from build123d import *

# Parameters (mm, degrees)
SKETCH1_W               = 203.2
SKETCH1_H               = 203.2
BOSS_EXTRUDE1_DEPTH     = 6.35
SKETCH2_W               = 44.45
SKETCH2_H               = 45.72
SKETCH2_H_2             = 50.8
CUT_EXTRUDE1_DEPTH      = 144.824345992
SKETCH3_R               = 2.54
SKETCH3_W               = 25.4
SKETCH3_H               = 25.4
CUT_EXTRUDE2_DEPTH      = 6.35
MIRROR2_COPY_1_SKETCH_R = 2.54
MIRROR2_COPY_1_SKETCH_W = 25.4
MIRROR2_COPY_1_SKETCH_H = 25.4
MIRROR2_COPY_1_DEPTH    = 6.35
SKETCH4_W               = 101.6
SKETCH4_H               = 93.98
SKETCH4_W_2             = 95.25
SKETCH4_H_2             = 87.63
BOSS_EXTRUDE2_DEPTH     = 152.4
SKETCH5_W               = 10
SKETCH5_H               = 10
SKETCH5_R               = 1.6
BOSS_EXTRUDE3_DEPTH     = 3.175
CUT_EXTRUDE3_REACH      = 246.393
SKETCH8_R               = 1.905
SKETCH9_W               = 6.35
SKETCH9_H               = 152.4
BOSS_EXTRUDE4_DEPTH     = 44.45
SKETCH12_W              = 3.175
SKETCH12_H              = 3.81
CUT_EXTRUDE4_DEPTH      = 152.4
SKETCH13_W              = 38.1
SKETCH13_H              = 3.81
CUT_EXTRUDE5_DEPTH      = 3.175
SKETCH14_W              = 6.35
SKETCH14_H              = 152.4
BOSS_EXTRUDE5_DEPTH     = 44.45
SKETCH15_W              = 3.175
SKETCH15_H              = 3.81
CUT_EXTRUDE6_DEPTH      = 152.4
SKETCH16_W              = 38.1
SKETCH16_H              = 3.81
CUT_EXTRUDE7_DEPTH      = 3.175
CUT_EXTRUDE8_REACH      = 211.454
SKETCH17_R              = 6.35
MIRROR5_OUTLINE_R       = 6.35
MIRROR5_DEPTH           = 6.35


# Read off the part's stored shape, not the designer's step: Mirror5
with BuildPart() as part:
    # Sketch1 → Boss-Extrude1 (new body)
    with BuildSketch(Plane(origin=(0, 0, 0), x_dir=(1, 0, 0), z_dir=(0, 1, 0))):
        Rectangle(SKETCH1_W, SKETCH1_H)
    extrude(amount=BOSS_EXTRUDE1_DEPTH)

    # Sketch2 → Cut-Extrude1 (cut, through all)
    with BuildSketch(Plane(origin=(0, 6.35, 0), x_dir=(1, 0, 0), z_dir=(0, 1, 0))):
        with Locations((0, 78.74)):
            Rectangle(SKETCH2_W, SKETCH2_H)
        with Locations((0, -76.2)):
            Rectangle(SKETCH2_W, SKETCH2_H_2)
    extrude(amount=-CUT_EXTRUDE1_DEPTH, mode=Mode.SUBTRACT)

    # Sketch3 → Cut-Extrude2 (cut)
    with BuildSketch(Plane(origin=(0, 6.35, 0), x_dir=(1, 0, 0), z_dir=(0, 1, 0))):
        with Locations(Location((-96.52, 76.2, 0), (0, 0, 270))):
            Circle(SKETCH3_R)
        with Locations(Location((-76.2, 96.52, 0), (0, 0, 270))):
            Circle(SKETCH3_R)
        with Locations(Location((-76.2, 55.88, 0), (0, 0, 270))):
            Circle(SKETCH3_R)
        with Locations(Location((-41.275, 96.52, 0), (0, 0, 270))):
            Circle(SKETCH3_R)
        with Locations(Location((-41.275, 55.88, 0), (0, 0, 90))):
            Circle(SKETCH3_R)
        with Locations((-41.148, 76.2)):
            Rectangle(SKETCH3_W, SKETCH3_H)
        with Locations((-76.2, 76.2)):
            Rectangle(SKETCH3_W, SKETCH3_H)
    cut_extrude2 = extrude(amount=-CUT_EXTRUDE2_DEPTH, mode=Mode.SUBTRACT)

    # Mirror1: Cut-Extrude2 across plane
    add(cut_extrude2.mirror(Plane(origin=(0, 0, 0), x_dir=(0, 0, 1), z_dir=(1, 0, 0))), mode=Mode.SUBTRACT)

    # Mirror2: Cut-Extrude2 across plane
    add(cut_extrude2.mirror(Plane.XY), mode=Mode.SUBTRACT)

    # Mirror2 copy 1 sketch → Mirror2 copy 1 (cut)
    with BuildSketch(Plane(origin=(0, 6.35, 0), x_dir=(-1, 0, 0), z_dir=(0, 1, 0))):
        with Locations(Location((-96.52, 76.2, 0), (0, 0, 270))):
            Circle(MIRROR2_COPY_1_SKETCH_R)
        with Locations(Location((-76.2, 96.52, 0), (0, 0, 270))):
            Circle(MIRROR2_COPY_1_SKETCH_R)
        with Locations(Location((-76.2, 55.88, 0), (0, 0, 270))):
            Circle(MIRROR2_COPY_1_SKETCH_R)
        with Locations(Location((-41.275, 96.52, 0), (0, 0, 270))):
            Circle(MIRROR2_COPY_1_SKETCH_R)
        with Locations(Location((-41.275, 55.88, 0), (0, 0, 90))):
            Circle(MIRROR2_COPY_1_SKETCH_R)
        with Locations((-41.148, 76.2)):
            Rectangle(MIRROR2_COPY_1_SKETCH_W, MIRROR2_COPY_1_SKETCH_H)
        with Locations((-76.2, 76.2)):
            Rectangle(MIRROR2_COPY_1_SKETCH_W, MIRROR2_COPY_1_SKETCH_H)
    extrude(amount=-MIRROR2_COPY_1_DEPTH, mode=Mode.SUBTRACT)

    # Sketch4 → Boss-Extrude2 (add)
    with BuildSketch(Plane(origin=(0, 6.35, 0), x_dir=(1, 0, 0), z_dir=(0, 1, 0))):
        with Locations((0, 2.54)):
            Rectangle(SKETCH4_W, SKETCH4_H)
        with Locations((0, 2.54)):
            Rectangle(SKETCH4_W_2, SKETCH4_H_2, mode=Mode.SUBTRACT)
    extrude(amount=BOSS_EXTRUDE2_DEPTH)

    # Sketch5 → Boss-Extrude3 (add)
    # profile 1 of 4: a face of its own
    with BuildSketch(Plane(origin=(50.8, 0, 0), x_dir=(0, 0, -1), z_dir=(1, 0, 0))):
        with Locations((-21.59, 93.98)):
            Rectangle(SKETCH5_W, SKETCH5_H)
        with Locations((-21.59, 93.98)):
            Circle(SKETCH5_R, mode=Mode.SUBTRACT)
    # profile 2 of 4: a face of its own
    with BuildSketch(Plane(origin=(50.8, 0, 0), x_dir=(0, 0, -1), z_dir=(1, 0, 0))):
        with Locations((26.67, 92.71)):
            Rectangle(SKETCH5_W, SKETCH5_H)
        with Locations((26.67, 92.71)):
            Circle(SKETCH5_R, mode=Mode.SUBTRACT)
    # profile 3 of 4: a face of its own
    with BuildSketch(Plane(origin=(50.8, 0, 0), x_dir=(0, 0, -1), z_dir=(1, 0, 0))):
        with Locations((-21.59, 11.43)):
            Rectangle(SKETCH5_W, SKETCH5_H)
        with Locations((-21.59, 11.43)):
            Circle(SKETCH5_R, mode=Mode.SUBTRACT)
    # profile 4 of 4: a face of its own
    with BuildSketch(Plane(origin=(50.8, 0, 0), x_dir=(0, 0, -1), z_dir=(1, 0, 0))):
        with Locations((26.67, 17.78)):
            Rectangle(SKETCH5_W, SKETCH5_H)
        with Locations((26.67, 17.78)):
            Circle(SKETCH5_R, mode=Mode.SUBTRACT)
    extrude(amount=BOSS_EXTRUDE3_DEPTH)

    # Sketch8 → Cut-Extrude3 (cut, up to next)
    with BuildSketch(Plane(origin=(53.975, 0, 0), x_dir=(0, 0, -1), z_dir=(1, 0, 0)), mode=Mode.PRIVATE) as cut_extrude3_sk1:
        with Locations((-21.59, 93.98)):
            Circle(SKETCH8_R)
    cut_extrude3_tool1 = extrude(cut_extrude3_sk1.sketch, amount=-CUT_EXTRUDE3_REACH, mode=Mode.PRIVATE) & part.part
    # Sketch8 → Cut-Extrude3 (cut, up to next)
    with BuildSketch(Plane(origin=(53.975, 0, 0), x_dir=(0, 0, -1), z_dir=(1, 0, 0)), mode=Mode.PRIVATE) as cut_extrude3_sk2:
        with Locations((26.67, 92.71)):
            Circle(SKETCH8_R)
    cut_extrude3_tool2 = extrude(cut_extrude3_sk2.sketch, amount=-CUT_EXTRUDE3_REACH, mode=Mode.PRIVATE) & part.part
    # Sketch8 → Cut-Extrude3 (cut, up to next)
    with BuildSketch(Plane(origin=(53.975, 0, 0), x_dir=(0, 0, -1), z_dir=(1, 0, 0)), mode=Mode.PRIVATE) as cut_extrude3_sk3:
        with Locations((-21.59, 11.43)):
            Circle(SKETCH8_R)
    cut_extrude3_tool3 = extrude(cut_extrude3_sk3.sketch, amount=-CUT_EXTRUDE3_REACH, mode=Mode.PRIVATE) & part.part
    # Sketch8 → Cut-Extrude3 (cut, up to next)
    with BuildSketch(Plane(origin=(53.975, 0, 0), x_dir=(0, 0, -1), z_dir=(1, 0, 0)), mode=Mode.PRIVATE) as cut_extrude3_sk4:
        with Locations((26.67, 17.78)):
            Circle(SKETCH8_R)
    cut_extrude3_tool4 = extrude(cut_extrude3_sk4.sketch, amount=-CUT_EXTRUDE3_REACH, mode=Mode.PRIVATE) & part.part
    add(cut_extrude3_tool1.solids().sort_by_distance((53.975, 93.98, 21.59))[0], mode=Mode.SUBTRACT)
    add(cut_extrude3_tool2.solids().sort_by_distance((53.975, 92.71, -26.67))[0], mode=Mode.SUBTRACT)
    add(cut_extrude3_tool3.solids().sort_by_distance((53.975, 11.43, 21.59))[0], mode=Mode.SUBTRACT)
    add(cut_extrude3_tool4.solids().sort_by_distance((53.975, 17.78, -26.67))[0], mode=Mode.SUBTRACT)

    # Sketch9 → Boss-Extrude4 (add)
    with BuildSketch(Plane(origin=(50.8, 0, 0), x_dir=(0, 0, -1), z_dir=(1, 0, 0))):
        with Locations((-41.275, 82.55)):
            Rectangle(SKETCH9_W, SKETCH9_H)
        with Locations((46.355, 82.55)):
            Rectangle(SKETCH9_W, SKETCH9_H)
    extrude(amount=BOSS_EXTRUDE4_DEPTH)

    # Sketch12 → Cut-Extrude4 (cut)
    with BuildSketch(Plane(origin=(0, 158.75, 0), x_dir=(1, 0, 0), z_dir=(0, 1, 0))):
        with Locations((90.4875, -40.005)):
            Rectangle(SKETCH12_W, SKETCH12_H)
    cut_extrude4 = extrude(amount=-CUT_EXTRUDE4_DEPTH, mode=Mode.SUBTRACT)

    # Sketch13 → Cut-Extrude5 (cut)
    with BuildSketch(Plane(origin=(0, 158.75, 0), x_dir=(1, 0, 0), z_dir=(0, 1, 0))):
        with Locations((69.85, -40.005)):
            Rectangle(SKETCH13_W, SKETCH13_H)
    cut_extrude5 = extrude(amount=-CUT_EXTRUDE5_DEPTH, mode=Mode.SUBTRACT)

    # Mirror3: Cut-Extrude4, Cut-Extrude5 across plane
    add(cut_extrude4.mirror(Plane(origin=(0, 0, -2.54), x_dir=(1, 0, 0), z_dir=(0, 0, -1))), mode=Mode.SUBTRACT)
    add(cut_extrude5.mirror(Plane(origin=(0, 0, -2.54), x_dir=(1, 0, 0), z_dir=(0, 0, -1))), mode=Mode.SUBTRACT)

    # Sketch14 → Boss-Extrude5 (add)
    with BuildSketch(Plane.ZY.offset(50.8)):
        with Locations((-46.355, 82.55)):
            Rectangle(SKETCH14_W, SKETCH14_H)
        with Locations((41.275, 82.55)):
            Rectangle(SKETCH14_W, SKETCH14_H)
    extrude(amount=BOSS_EXTRUDE5_DEPTH)

    # Sketch15 → Cut-Extrude6 (cut)
    with BuildSketch(Plane(origin=(0, 158.75, 0), x_dir=(1, 0, 0), z_dir=(0, 1, 0))):
        with Locations((-90.4875, -40.005)):
            Rectangle(SKETCH15_W, SKETCH15_H)
    cut_extrude6 = extrude(amount=-CUT_EXTRUDE6_DEPTH, mode=Mode.SUBTRACT)

    # Sketch16 → Cut-Extrude7 (cut)
    with BuildSketch(Plane(origin=(0, 158.75, 0), x_dir=(1, 0, 0), z_dir=(0, 1, 0))):
        with Locations((-69.85, -40.005)):
            Rectangle(SKETCH16_W, SKETCH16_H)
    cut_extrude7 = extrude(amount=-CUT_EXTRUDE7_DEPTH, mode=Mode.SUBTRACT)

    # Mirror4: Cut-Extrude6, Cut-Extrude7 across plane
    add(cut_extrude6.mirror(Plane(origin=(0, 0, -2.54), x_dir=(1, 0, 0), z_dir=(0, 0, -1))), mode=Mode.SUBTRACT)
    add(cut_extrude7.mirror(Plane(origin=(0, 0, -2.54), x_dir=(1, 0, 0), z_dir=(0, 0, -1))), mode=Mode.SUBTRACT)

    # Sketch17 → Cut-Extrude8 (cut, up to next)
    with BuildSketch(Plane(origin=(0, 6.35, 0), x_dir=(1, 0, 0), z_dir=(0, 1, 0)), mode=Mode.PRIVATE) as cut_extrude8_sk1:
        with Locations(Location((-76.2, -16.51, 0), (0, 0, 270))):
            Circle(SKETCH17_R)
    cut_extrude8_tool1 = extrude(cut_extrude8_sk1.sketch, amount=-CUT_EXTRUDE8_REACH, mode=Mode.PRIVATE) & part.part
    # Sketch17 → Cut-Extrude8 (cut, up to next)
    with BuildSketch(Plane(origin=(0, 6.35, 0), x_dir=(1, 0, 0), z_dir=(0, 1, 0)), mode=Mode.PRIVATE) as cut_extrude8_sk2:
        with Locations(Location((-76.2, 21.59, 0), (0, 0, 90))):
            Circle(SKETCH17_R)
    cut_extrude8_tool2 = extrude(cut_extrude8_sk2.sketch, amount=-CUT_EXTRUDE8_REACH, mode=Mode.PRIVATE) & part.part
    # Sketch17 → Cut-Extrude8 (cut, up to next)
    with BuildSketch(Plane(origin=(0, 6.35, 0), x_dir=(1, 0, 0), z_dir=(0, 1, 0)), mode=Mode.PRIVATE) as cut_extrude8_sk3:
        with Locations(Location((-28.575, 27.305, 0), (0, 0, 270))):
            Circle(SKETCH17_R)
    cut_extrude8_tool3 = extrude(cut_extrude8_sk3.sketch, amount=-CUT_EXTRUDE8_REACH, mode=Mode.PRIVATE) & part.part
    # Sketch17 → Cut-Extrude8 (cut, up to next)
    with BuildSketch(Plane(origin=(0, 6.35, 0), x_dir=(1, 0, 0), z_dir=(0, 1, 0)), mode=Mode.PRIVATE) as cut_extrude8_sk4:
        with Locations(Location((28.575, -22.225, 0), (0, 0, 270))):
            Circle(SKETCH17_R)
    cut_extrude8_tool4 = extrude(cut_extrude8_sk4.sketch, amount=-CUT_EXTRUDE8_REACH, mode=Mode.PRIVATE) & part.part
    add(cut_extrude8_tool1.solids().sort_by_distance((-76.2, 6.35, 16.51))[0], mode=Mode.SUBTRACT)
    add(cut_extrude8_tool2.solids().sort_by_distance((-76.2, 6.35, -21.59))[0], mode=Mode.SUBTRACT)
    add(cut_extrude8_tool3.solids().sort_by_distance((-28.575, 6.35, -27.305))[0], mode=Mode.SUBTRACT)
    add(cut_extrude8_tool4.solids().sort_by_distance((28.575, 6.35, 22.225))[0], mode=Mode.SUBTRACT)

    # Mirror5 outline → Mirror5 (cut)
    with BuildSketch(Plane(origin=(0, 0, 0), x_dir=(1, 0, 0), z_dir=(0, 1, 0))):
        with Locations((76.2, 21.59)):
            Circle(MIRROR5_OUTLINE_R)
        with Locations((76.2, -16.51)):
            Circle(MIRROR5_OUTLINE_R)
    extrude(amount=MIRROR5_DEPTH, mode=Mode.SUBTRACT)


solid = part.part
Source: CAD feature listing. Evaluate the final solid. Frame: model axes, mm. A direction names the side the tool comes from. Round coordinates to 2 decimals unless told otherwise and drop trailing zeros. Loops run counter-clockwise (first coordinate to the right, second up) from the corner with the lowest first, then second, coordinate; pieces in that order, holes last.
Q1. Access query for faces 4 (the face through (0, 3, -55.88)), 5 (the face through (76, 3, 63.5)), 6 (the face through (90, 105, -46.99)), 7 (the face through (22.225, 3, 77)). Directions: +Z, -Z, +X, -X, +Y, -Y. A direction counts if a zero-diameter tool reaches every point of the face in a straight line with its end or side. Return the directions, or none.
Q2. Mould query, pull axis Z, two halves, no side actions, for faces 1 (the face through (-95.25, 84, 41)), 2 (the face through (-1, 6.35, -3)), 3 (the face through (61, 3, 101.6)). Classes: pulls with the +Z half, pulls with the -Z half, needs draft (parallel to the pull), parting line crosses it, or undercut.
Q3. First-contact query: P1, Ø3, axis at x = 24, z = 66.5, coming from the +Y side; P2, Ø5, axis at y = 96, z = 0.5, coming from the -X side; P3, Ø4, axis at y = 111, z = 40.5, coming from the -X side; P4, Ø12, axis at x = 40, z = 75.5, coming from the +Y side. Flat tips, straight axial feed; report the tip coordinate or a pass-through.
Q4. Ray query, line 1 (Z direction, x = -96, y = 2); line 2 (Z direction, x = -6, y = 132.5) (3 decimals); line 3 (X direction, y = 114, z = -36.5) (3 decimals). Return the intervals inside material, ascending.
Q5. Section B-B, the plane z = 7.5. Return loops of the section in (x, y) (3 decimals), plus the area to 3 significant figures.
Solutions:
1. face 4: -Z, +Y, -Y
1. face 5: +Y, -Y
1. face 6: +Y
1. face 7: +Z, +Y, -Y
2. face 1: needs draft
2. face 2: undercut
2. face 3: pulls with the +Z half
3. P1: stops at y = 6.35
3. P2: stops at x = -50.8
3. P3: stops at x = -95.25
3. P4: passes through
4. line 1: z = -101.6 to -78.69, -73.71 to 73.71, 78.69 to 101.6
4. line 2: z = -49.53 to -46.355, 41.275 to 44.45
4. line 3: x = -50.8 to -47.625, 47.625 to 50.8
5. outline: (-101.6, 0) - (101.6, 0) - (101.6, 6.35) - (50.8, 6.35) - (50.8, 158.75) - (47.625, 158.75) - (47.625, 6.35) - (-47.625, 6.35) - (-47.625, 158.75) - (-50.8, 158.75) - (-50.8, 6.35) - (-101.6, 6.35) - close
5. area: 2,260 mm2
